Geometry: final body of the model. Coordinates: model frame, mm. A direction names the side the tool comes from. Round coordinates to 2 decimals unless told otherwise and drop trailing zeros. Loops run counter-clockwise (first coordinate to the right, second up) from the corner with the lowest first, then second, coordinate; pieces in that order, holes last. Notation, with made-up numbers: (19.5, 32) - (46.5, 32) arc R29 cw to (46.5, 62) - close; hole circle Ø4 at (54.5, -8.75). An arc over 180 degrees is marked (long way). Answer as a JSON object with one key per item and string values. Group by question number.
Item 1: Reachability of faces 1 (the face through (0, 3.3, 0.1)), 2 (the face through (-6, -2, 2)), 3 (the face through (-4.411, -1.268, -2.155)) from +Z, -Z, +X, -X, +Y, -Y: full face, straight path, thin tool, end or side. Return the list, or none.
Item 2: Draft query along Z for faces 4 (the face through (-4.411, 1.268, 2.155)), 5 (the face through (22, -3, 0)), 6 (the face through (45, 0, 0)). Return one class per face: released by +Z, released by -Z, zero draft, split by the parting line, or undercut.
Item 3: Line query: line 1 (Z direction, x = 8, y = 0); line 2 (X direction, y = -3, z = 1.75); line 3 (Y direction, x = -3.5, z = -2.5). Output: solid intervals per line, ascending.
Item 4: Section A-A (x = 27). Return the cut outline in (y, z), plus the area to 3 significant figures.
Item 5: First-contact query: pin 1 (3 mm diameter, centred on x = 25, y = -4, fed in from +Z); pin 2 (5 mm diameter, centred on x = 17.5, y = -1, fed in from +Z). Flat tips, straight axial feed; report the tip coordinate or a pass-through.
Autodesk Inventor part; units mm, degrees
ref_plane "Work Plane1" through (29, 0, 0) normal (0, -1, 0) x (1, 0, 0)
ref_plane "YZ Plane" through (0, 0, 0) normal (1, 0, 0) x (0, 1, 0)
ref_plane "XZ Plane" through (0, 0, 0) normal (0, 1, 0) x (-1, 0, 0)
sketch "Sketch1" plane through (0, 0, 0) normal (0, 0, 1) x (1, 0, 0)
  line L0 (-1.3333, 0) -> (45, 0)
  line L1 (45, 0) -> (45, 3)
  line L2 (45, 3) -> (21, 3)
  line L3 (21, 3) -> (20.3864, 3)
  line L4 (20.3864, 3) -> (0, 3)
  line L5 (0, 3) -> (0, 5)
  line L6 (0, 5) -> (-6, 5)
  line L7 (-6, 5) -> (-6, 2.8868)
  line L8 (-6, 2.8868) -> (-3, 2.8868)
  line L9 (-3, 2.8868) -> (-1.3333, 0)
  line L10 (-11.1, 0) -> (60.3, 0)
  line L11 (0, -0.5) -> (0, 6.5)
  line L12 (21, 3) -> (0, 3) construction
  dimension "d1" = 24
  dimension "d2" = 0.6136
  dimension "d3" = 6
  dimension "d4" = 3
  dimension "d5" = 60
  dimension "d6" = 6
  dimension "d7" = 6
  dimension "d8" = 5.7735
  dimension "d9" = 10
  dimension "d26" = 45
revolve "Body" add sketch "Sketch1" angle 360 about axis through (-1.3333, 0, 0) along (1, 0, 0)
sketch "Sketch2" plane through (-6, 0, 0) normal (-1, 0, 0) x (0, 0, 1)
  circle A0 centre (0, 0) radius 2.8868
  line L0 (0, -6) -> (0, 8)
  line L1 (-6, 0) -> (8, 0)
  line L2 (2.8868, 0) -> (1.4434, -2.5)
  line L3 (1.4434, -2.5) -> (-1.4434, -2.5)
  line L4 (-1.4434, -2.5) -> (-2.8868, 0)
  line L5 (-2.8868, 0) -> (-1.4434, 2.5)
  line L6 (-1.4434, 2.5) -> (1.4434, 2.5)
  line L7 (1.4434, 2.5) -> (2.8868, 0)
extrude "Slot" add sketch "Sketch2" against normal up to next contours L7 A0 | A0 L2 | L6 L0 A0 | A0 L0 L3 | L0 L6 A0 | A0 L3 L0 | L4 A0 | A0 L5
fillet "Fillet1" radius 0.6 1 edges at (-6, -5, 0)
thread "Thread"
chamfer "Chamfer1" distance 0.6135 distance2 0.6135 1 edges at (45, -3, 0) measured on face at (45, -0.5525, -1.8157)
ref_plane "Work Plane1" through (29, 0, 0) normal (0, -1, 0) x (1, 0, 0)
equation "\"d1\" = GEL"
equation "\"d3\" = KOH"
equation "\"d4\" = INTI"
equation "\"d6\" = GD"
equation "\"d7\" = BDM"
equation "\"d8\" = 1.1547 * SW"
equation "\"d9\" = KOD"
equation "\"d26\" = NLG"
equation "\"d17\" = RR"
equation "\"d13\" = GEL"
equation "\"d15\" = -0.5 * SPD + 0.5 * GD"
equation "\"d16\" = GUL"
equation "\"GD\" = 6"
equation "\"NLG\" = 45"
equation "\"GEL\" = 24"
equation "\"KOD\" = 10"
equation "\"KOH\" = 6"
equation "\"INTI\" = 3"
equation "\"GAL\" = 0.61345 * PTC"
equation "\"GUL\" = 0.61345 * PTC"
equation "\"BDM\" = NND"
equation "\"SW\" = 5"
equation "\"RR\" = 0.6"
equation "\"SPD\" = NND - 1.2269 * PTC"
equation "\"TOA\" = 30deg"
equation "\"GD1\" = THREADDIA - 1.2269 * PTC"
equation "\"THREADDIA\" = 6"
equation "\"FAWI\" = 45deg"
equation "\"PTC\" = 1"
equation "\"NND\" = 6"
equation "\"E0\" = 1.155 * SW"
properties part number "100011" material "Steel, Mild"
Values:
{
 "1": {"face 1": "+X", "face 2": "+Z, -Z, -X, +Y, -Y", "face 3": "-X"},
 "2": {"face 4": "undercut", "face 5": "split by the parting line", "face 6": "zero draft"},
 "3": {"line 1": "z = -3 to 3", "line 2": "x = -6 to 0", "line 3": "y = -4.33 to -0.67, 0.67 to 4.33"},
 "4": {"outline": "circle Ø6 at (0, 0)", "area": "28.3 mm^2"},
 "5": {"pin 1": "stops at z = 1.66", "pin 2": "stops at z = 3"}
}
